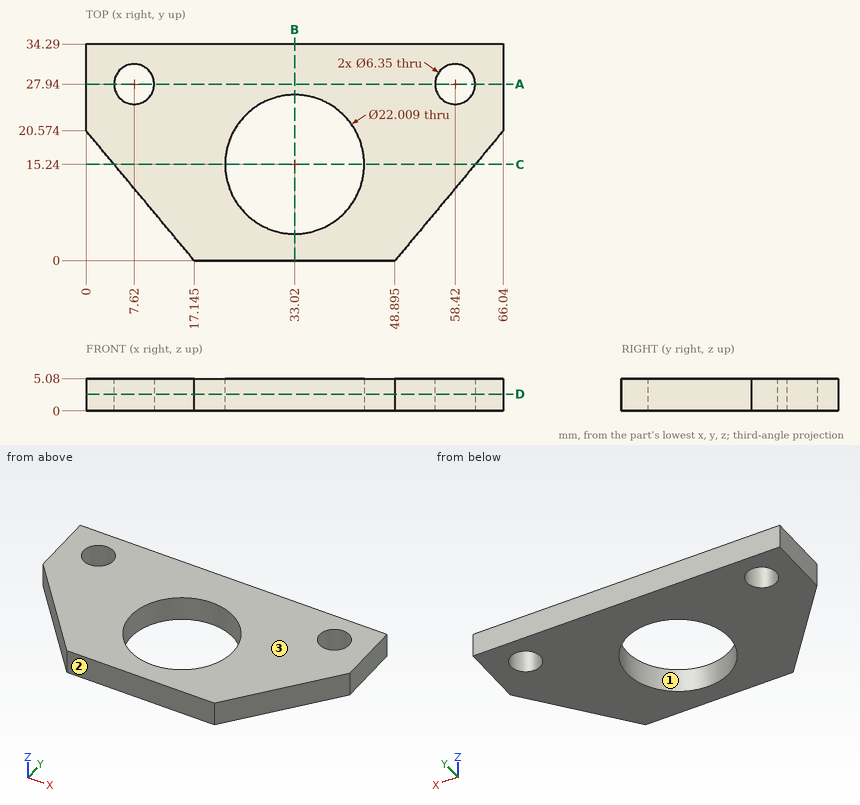
Job drawing, mm, ordinate dimensions from the low corner. One solid piece. Round coordinates to 2 decimals unless told otherwise and drop trailing zeros. Write each loop counter-clockwise with the first axis right and the second up, starting at its lowest first coordinate (ties: lowest second). Pieces come first, ordered by that corner, then holes.
1) Band-saw the part on D-D, the plane z = 2.65. Give the number of separate pieces and of enclosed holes in the cut face, and give its area (3 significant figures).
2) Drill centre lines: probe 1 along X at (y, z) = (29.5, 3.35) (1 decimal); probe 2 along X at (y, z) = (28.5, 0.3) (1 decimal); probe 3 along Y at (x, z) = (33.02, 3.75). Where is each one in solid material? Low to high.
3) Band-saw the part on A-A, the plane y = 27.94. List the corners of the cut face in (x, z) (3 decimals), and give its area (3 significant figures).
4) Pin check, flat tips, straight feed: pin 1 (2 mm diameter, centred on y = 23, z = 3, fed in from -X); pin 2 (13 mm diameter, centred on x = 33.02, y = 15.24, fed in from +Z); pin 3 (2 mm diameter, centred on x = 55, z = 1, fed in from -Y). Stop position of each tip, or through.
5) Band-saw the part on B-B, the plane x = 33.02. List the corners of the cut face in (y, z).
6) Band-saw the part on C-C, the plane y = 15.24. List the corners of the cut face in (x, z) (1 decimal).
7) Mould opens along Y. For the marked faces 1, 2 and 3 say: +Y half, -Y half, draft (parallel to the pull), parting line (faces both ways), or undercut.
Ans:
1. separate pieces: 1
1. enclosed holes: 3
1. area: 1,470 mm2
2. probe 1: x = 0 to 4.9, 10.4 to 55.7, 61.2 to 66
2. probe 2: x = 0 to 4.5, 10.7 to 55.3, 61.5 to 66
2. probe 3: y = 0 to 4.24, 26.24 to 34.29
3. outline: (0, 0) - (4.445, 0) - (4.445, 5.08) - (0, 5.08) - close; (10.795, 0) - (55.245, 0) - (55.245, 5.08) - (10.795, 5.08) - close; (61.595, 0) - (66.04, 0) - (66.04, 5.08) - (61.595, 5.08) - close
3. area: 271 mm2
4. pin 1: stops at x = 0
4. pin 2: passes through
4. pin 3: stops at y = 6.13
5. outline: (0, 0) - (4.24, 0) - (4.24, 5.08) - (0, 5.08) - close; (26.24, 0) - (34.29, 0) - (34.29, 5.08) - (26.24, 5.08) - close
6. outline: (4.4, 0) - (22, 0) - (22, 5.1) - (4.4, 5.1) - close; (44, 0) - (61.6, 0) - (61.6, 5.1) - (44, 5.1) - close
7. face 1: undercut
7. face 2: -Y half
7. face 3: draft
